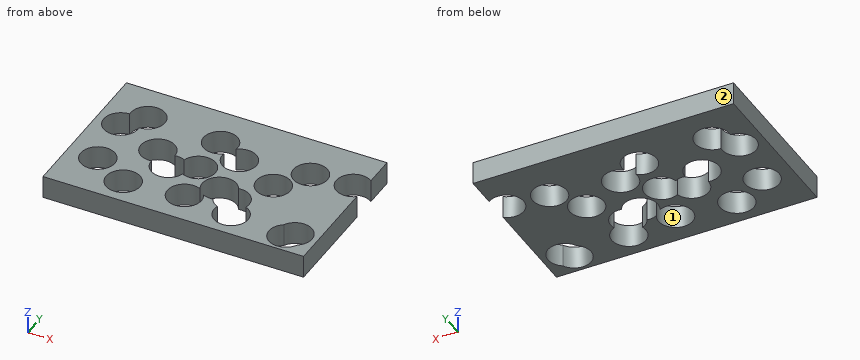
from build123d import *

# Parameters (mm, degrees)
SKICA1_W                 = 114.49904762
SKICA1_H                 = 70.201904762
P_IDAT_VYSUNUT_M1_DEPTH  = 10
ODEBRAT_VYSUNUT_M1_REACH = 69.894
SKICA2_R                 = 7.5


with BuildPart() as part:
    # Skica1 → Přidat vysunutím1 (new body)
    with BuildSketch(Plane.XY):
        Rectangle(SKICA1_W, SKICA1_H)
    extrude(amount=P_IDAT_VYSUNUT_M1_DEPTH)

    # Skica2 → Odebrat vysunutím1 (cut, up to next)
    with BuildSketch(Plane(origin=(0, 0, 0), x_dir=(-1, 0, 0), z_dir=(0, 0, -1)), mode=Mode.PRIVATE) as odebrat_vysunut_m1_sk1:
        with Locations((-44.884870965, -26.225697914)):
            Circle(SKICA2_R)
    odebrat_vysunut_m1_tool1 = extrude(odebrat_vysunut_m1_sk1.sketch, amount=-ODEBRAT_VYSUNUT_M1_REACH, mode=Mode.PRIVATE) & part.part
    odebrat_vysunut_m1 = odebrat_vysunut_m1_tool1.solids().sort_by_distance((44.884871, -26.225698, 0))[0]
    add(odebrat_vysunut_m1, mode=Mode.SUBTRACT)

    # Skica-pole1: Odebrat vysunutím1 at 17 more places
    with Locations((-10.431632, 40.559072, 0), (-47.510307, 5.535631, 0), (-91.431484, 36.089944, 0), (-19.820495, 27.327921, 0), (-29.869712, 11.905495, 0), (-39.296811, 36.089944, 0), (-51.262991, 43.110266, 0), (-73.00145, 2.810383, 0), (-62.00138, 19.782901, 0), (-70.543611, 27.327921, 0), (-51.262991, 24.48943, 0), (-37.6102, 15.915325, 0), (2.492308, 2.810383, 0), (7.770749, 41.83746, 0), (-25.552545, 2.810383, 0), (-88.893218, 11.905495, 0), (-84.014078, 44.651823, 0)):
        add(odebrat_vysunut_m1, mode=Mode.SUBTRACT)


solid = part.part
Could you check a few things on this model? Use its own coordinates, in mm. Face numbers are marked on the shaded views. Give positions to 0.01 mm unless a question says otherwise; leave off trailing zeros. Loops run counter-clockwise (first coordinate to the right, second up) from the corner with the lowest first, then second, coordinate; pieces in that order, holes last. Notation, with made-up numbers: M 83,39.5 L 107,39.5 A27 ccw 107,75.5 Z; hole C -33.75,60.25 d5. An arc over 180 degrees is marked long. Answer as a JSON object with one key per item and string values.
Q1. If I drill on probe 1 along Y at (x, z) = (31, 8.5); probe 2 along Y at (x, z) = (-30.5, 6); probe 3 along X at (y, z) = (3, 8.5), over which ranges is the centre line in solid material (lowest first)? Write a range as [from, to].
Values found:
{"probe 1": "y = [-35.1, -3.48], [5.69, 7.68], [20.99, 35.1]", "probe 2": "y = [-35.1, -30.53], [-16.3, -4.63], [6.83, 35.1]", "probe 3": "x = [-57.25, -49.57], [-43.52, -32.91], [-18.4, -12.19], [-0.56, 2.57], [8.61, 17.81], [32.32, 57.25]"}
Q2. If we mould it in two halves opening along X, with no side actions, what happens to the marked faces 1 and 2? For each: pulls with the +X half, pulls with the -X half, needs draft (parallel to the pull), parting line crosses it, or undercut.
Values found:
{"face 1": "undercut", "face 2": "needs draft"}
Q3. For P1, Ø13.5, axis at x = 52.66, y = 15.61, coming from the +Z side, with a flat end and sliding along its axis, tell me the tip position at first contact or that it passes through.
Values found:
{"P1": "passes through"}
Q4. Suppose I cut it at C-C, the plane z = 4.5. State how many separate pieces and enclosed holes the cut face has, plus the area to 3 significant figures.
Values found:
{"separate pieces": "1", "enclosed holes": "9", "area": "5,170 mm²"}
Q5. Suppose I cut it at B-B, the plane y = -25. List the corners of the cut face in (x, z) for me.
Values found:
{"outline": "M -57.25,0 L -35.45,0 L -35.45,10 L -57.25,10 Z; M -20.79,0 L -8.76,0 L -8.76,10 L -20.79,10 Z; M 3.51,0 L 12,0 L 12,10 L 3.51,10 Z; M 26.66,0 L 37.49,0 L 37.49,10 L 26.66,10 Z; M 54.71,0 L 57.25,0 L 57.25,10 L 54.71,10 Z"}
Q6. Suppose I cut it at D-D, the plane x = 35. List the corners of the cut face in (y, z) for me.
Values found:
{"outline": "M -35.1,0 L 6.85,0 L 6.85,10 L -35.1,10 Z; M 21.81,0 L 35.1,0 L 35.1,10 L 21.81,10 Z"}
Q7. Suppose I cut it at A-A, the plane x = 6.5. List the corners of the cut face in (y, z) for me, plus the area to 3 significant figures.
Values found:
{"outline": "M -35.1,0 L -17.77,0 L -17.77,10 L -35.1,10 Z; M -2.85,0 L 2.42,0 L 2.42,10 L -2.85,10 Z; M 17.31,0 L 35.1,0 L 35.1,10 L 17.31,10 Z", "area": "404 mm²"}
